```python
from build123d import *

# Parameters (mm, degrees)
F1_DEPTH = 3
F2_R     = 1.5
F3_R     = 3


with BuildPart() as f1:
    # F0 (on Top) → F1 (new body)
    with BuildSketch(Plane.XY):
        with BuildLine():
            Line((-15, 21), (-22, 0))
            Line((-22, 0), (22, 0))
            Line((22, 0), (16.046474, 17.860578))
            Line((16.046474, 17.860578), (-1.966555, 32.446361))
            ThreePointArc((-1.966555, 32.446361), (-1.345389, 37.695559), (3.125, 34.875))
            ThreePointArc((3.125, 34.875), (2.94577, 33.831897), (2.428639, 32.908445))
            Line((2.428639, 32.908445), (14.21061, 23.368169))
            Line((14.21061, 23.368169), (0, 66))
            Line((0, 66), (-13.944539, 24.166384))
            Line((-13.944539, 24.166384), (-2.428639, 14.841555))
            ThreePointArc((-2.428639, 14.841555), (1.043103, 15.82077), (3.125, 12.875))
            ThreePointArc((3.125, 12.875), (1.345389, 10.054441), (-1.966555, 10.446361))
            Line((-1.966555, 10.446361), (-15, 21))
        make_face()
    extrude(amount=F1_DEPTH)

    # F2
    f2_edges = [f1.edges().sort_by_distance(p)[0] for p in [
        (-22, 0, 1.5),
        (22, 0, 1.5),
        (14.21061, 23.368169, 1.5),
        (0, 66, 1.5),
        (-15, 21, 1.5),
    ]]
    fillet(f2_edges, radius=F2_R)

    # F3
    f3_edges = [f1.edges().sort_by_distance(p)[0] for p in [
        (-13.944539, 24.166384, 1.5),
        (16.046474, 17.860578, 1.5),
    ]]
    fillet(f3_edges, radius=F3_R)


solid = f1.part
```
Geometry check sheet. Reference: the model listing, model coordinates, mm. A direction names the side the tool comes from. Round coordinates to 2 decimals unless told otherwise and drop trailing zeros. Loops run counter-clockwise (first coordinate to the right, second up) from the corner with the lowest first, then second, coordinate; pieces in that order, holes last. Notation, with made-up numbers: (88, 44.5) - (129, 44.5) arc R35 ccw to (129, 81.5) - close; hole circle Ø7 at (-29, 35). An arc over 180 degrees is marked (long way). Write each question's results on one line, items separated by ' | '. Start each with the question number.
Q1. Cross-section at D-D on y = 58.5. Enter the section's corners in (x, z).
Q2. Cross-section at B-B on x = -11. Enter the section's corners in (y, z), and give its area (3 significant figures).
Q3. Cross-section at C-C on x = 0. Enter the section's corners in (y, z).
Q4. Release check for a two-part mould opening along Y. For faces 3 (the cylindrical face through (0.026, 62.756, 1.521)), 4 (the flat face through (6.27, 29.8, 1.48)), 5 (the cylindrical face through (21.124, 0.607, 1.521)) record: +Y half, -Y half, draft (parallel to the pull), parting line (faces both ways), or undercut.
Q5. Cross-section at A-A on z = 1.7. Enter the section's corners in (x, y) (3 decimals).
Q6. Access from +Z, -Z, +X, -X, +Y, -Y to the whole of each face (thin tool, end or side, straight path). Record for faces 1 (the flat face through (7, 45, 1)), 2 (the flat face through (-7.563, 14.978, 1.479)).
Q7. Thickness scan on line 1 (Y direction, x = 0, z = 1.45); line 2 (X direction, y = 32, z = 0.7); line 3 (X direction, y = 28, z = 0.75). Record the ranges inside material, lowest first. Write a range as [from, to].
Answers below:
1) outline: (-2.5, 0) - (2.5, 0) - (2.5, 3) - (-2.5, 3) - close
2) outline: (0, 0) - (17.76, 0) - (17.76, 3) - (0, 3) - close; (21.78, 0) - (33, 0) - (33, 3) - (21.78, 3) - close | area: 86.9 mm²
3) outline: (0, 0) - (9.75, 0) - (9.75, 3) - (0, 3) - close; (16, 0) - (30.85, 0) - (30.85, 3) - (16, 3) - close; (38, 0) - (62.76, 0) - (62.76, 3) - (38, 3) - close
4) face 3: +Y half | face 4: undercut | face 5: parting line
5) outline: (-21.342, 1.974) arc R1.5 ccw to (-19.919, 0) - (19.919, 0) arc R1.5 ccw to (21.342, 1.974) - (16.324, 17.029) arc R3 ccw to (15.365, 18.412) - (-1.967, 32.446) arc R3.125 cw (long way) to (3.125, 34.875) arc R3.125 cw to (2.429, 32.908) - (10.22, 26.6) arc R1.5 ccw to (12.587, 28.24) - (1.423, 61.731) arc R1.5 ccw to (-1.423, 61.731) - (-13.287, 26.138) arc R3 ccw to (-12.329, 22.858) - (-2.429, 14.842) arc R3.125 cw (long way) to (-1.967, 10.446) - (-13.318, 19.638) arc R1.5 ccw to (-15.685, 18.946) - close
6) face 1: +Z, -Z, +X, +Y | face 2: +Z, -Z
7) line 1: y = [0, 9.75], [16, 30.85], [38, 62.76] | line 2: x = [-11.33, -1.42], [3.55, 11.33] | line 3: x = [-12.67, 3.52], [8.49, 12.65]
